```python
from build123d import *

# Parameters (mm, degrees)
BOSS_EXTRUDE1_DEPTH = 5.969
SKETCH2_R           = 1.75
SKETCH2_R_2         = 1.750000056
CUT_EXTRUDE1_DEPTH  = 5.969


with BuildPart() as part:
    # Sketch1 → Boss-Extrude1 (new body)
    with BuildSketch(Plane(origin=(0, 0, 0), x_dir=(1, 0, 0), z_dir=(0, 1, 0))):
        Polygon((3.909848904, 42), (0, 38.007654129), (0, 3.951224), (3.951224, 0), (38.048776, 0), (42, 3.951224), (42, 38.054127921), (38.043254173, 42), align=None)
    extrude(amount=BOSS_EXTRUDE1_DEPTH)

    # Sketch2 → Cut-Extrude1 (cut)
    with BuildSketch(Plane(origin=(0, 5.969, 0), x_dir=(1, 0, 0), z_dir=(0, 1, 0))):
        with Locations(Location((5.5, 36.479439065, 0), (0, 0, 270))):
            Circle(SKETCH2_R)
        with Locations(Location((36.5, 36.479439065, 0), (0, 0, 270))):
            Circle(SKETCH2_R_2)
        with Locations(Location((36.5, 5.479439065, 0), (0, 0, 270))):
            Circle(SKETCH2_R_2)
        with Locations(Location((5.5, 5.479439065, 0), (0, 0, 270))):
            Circle(SKETCH2_R_2)
    extrude(amount=-CUT_EXTRUDE1_DEPTH, mode=Mode.SUBTRACT)


solid = part.part
```
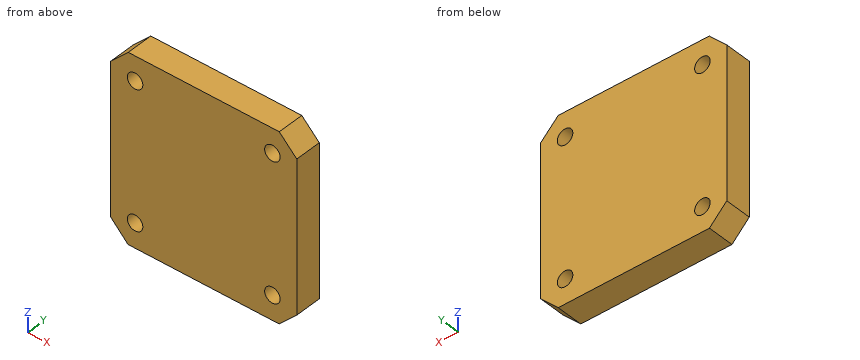
The listing builds one solid part. Answer for the finished solid, in the listing's coordinates (mm). Round coordinates to 2 decimals unless told otherwise and drop trailing zeros. Write each loop counter-clockwise with the first axis right and the second up, starting at its lowest first coordinate (ties: lowest second). Pieces come first, ordered by that corner, then holes. Notation, with made-up numbers: (15.25, 47.5) -> (39.25, 47.5) arc R25 ccw to (39.25, 72.5) -> close; hole circle Ø9 at (-5, -8.75). An arc over 180 degrees is marked (long way). Answer as a JSON object with one key per item and string values. Group by question number.
Q1. Section C-C (z = -6) is taken. Write down the section's boundary in (x, y), plus the area to 3 significant figures.
Q2. This flat-tipped pin is pushed along its axis until it touches: pin 1 Ø3 at (x, z) = (5.5, -5.48) entering from +Y. Where does it stop, or does it pass through?
Q3. Section A-A (x = 5.5) is taken. Write down the section's boundary in (y, z).
Q4. Section B-B (y = 0.5) is taken. Write down the section's boundary in (x, z).
Q5. Section D-D (x = 39) is taken. Write down the section's boundary in (y, z).
Q6. Straight lines are drawn through the part: line 1 along Z through (x, y) = (4, 0.4); line 2 along X through (y, z) = (5.6, -6.5); line 3 along Z through (x, y) = (5, 2.1). For each, find the intervals that lie inside material, in ascending order.
Check values:
{
 "1": {"outline": "(0, 0) -> (3.83, 0) -> (3.83, 5.97) -> (0, 5.97) -> close; (7.17, 0) -> (34.83, 0) -> (34.83, 5.97) -> (7.17, 5.97) -> close; (38.17, 0) -> (42, 0) -> (42, 5.97) -> (38.17, 5.97) -> close", "area": "211 mm^2"},
 "2": {"pin 1": "through"},
 "3": {"outline": "(0, -42) -> (5.97, -42) -> (5.97, -38.23) -> (0, -38.23) -> close; (0, -34.73) -> (5.97, -34.73) -> (5.97, -7.23) -> (0, -7.23) -> close; (0, -3.73) -> (5.97, -3.73) -> (5.97, 0) -> (0, 0) -> close"},
 "4": {"outline": "(0, -38.01) -> (3.91, -42) -> (38.04, -42) -> (42, -38.05) -> (42, -3.95) -> (38.05, 0) -> (3.95, 0) -> (0, -3.95) -> close; hole circle Ø3.5 at (5.5, -36.48); hole circle Ø3.5 at (5.5, -5.48); hole circle Ø3.5 at (36.5, -36.48); hole circle Ø3.5 at (36.5, -5.48)"},
 "5": {"outline": "(0, -41.05) -> (5.97, -41.05) -> (5.97, -0.95) -> (0, -0.95) -> close"},
 "6": {"line 1": "-42 to -37.38, -35.58 to -6.38, -4.58 to 0", "line 2": "0 to 4.08, 6.92 to 35.08, 37.92 to 42", "line 3": "-42 to -38.16, -34.8 to -7.16, -3.8 to 0"}
}
